Read the model definition and answer for the solid it produces. Units are mm, in the model's axes. Coordinates: 2 decimals unless noted, no trailing zeros. Write each loop counter-clockwise with the first axis right and the second up, starting at its lowest first coordinate (ties: lowest second). Pieces come first, ordered by that corner, then holes. Notation, with made-up numbers: (71, 61) - (101, 61) arc R22 cw to (101, 78) - close; hole circle Ø11 at (37.25, 31). An arc over 180 degrees is marked (long way). Use a Markdown table: item, result.
from build123d import *

# Parameters (mm, degrees)
SKETCH_1_W          = 381
SKETCH_1_H          = 110
EXTRUDE_1_DEPTH     = 5
SKETCH_2_R          = 2
CUT_EXTRUDE_1_DEPTH = 5
CUT_EXTRUDE_2_DEPTH = 5
SKETCH_6_R          = 1.5
CUT_EXTRUDE_3_DEPTH = 5
CUT_EXTRUDE_4_DEPTH = 10
FILLET_1_R          = 10


with BuildPart() as part:
    # 草图1 → 凸台-拉伸1 (new body)
    with BuildSketch(Plane.XY):
        with Locations((190.5, 55)):
            Rectangle(SKETCH_1_W, SKETCH_1_H)
    extrude(amount=EXTRUDE_1_DEPTH)

    # 草图2 → 切除-拉伸1 (cut)
    with BuildSketch(Plane.XY.offset(5)):
        with Locations((3.5, 105)):
            Circle(SKETCH_2_R)
        with Locations((3.5, 55)):
            Circle(SKETCH_2_R)
        with Locations((3.5, 5)):
            Circle(SKETCH_2_R)
        with Locations((377.5, 105)):
            Circle(SKETCH_2_R)
        with Locations((377.5, 55)):
            Circle(SKETCH_2_R)
        with Locations((377.5, 5)):
            Circle(SKETCH_2_R)
        with Locations((91.65, 105)):
            Circle(SKETCH_2_R)
        with Locations((91.65, 55)):
            Circle(SKETCH_2_R)
        with Locations((91.65, 5)):
            Circle(SKETCH_2_R)
        with Locations((289.35, 105)):
            Circle(SKETCH_2_R)
        with Locations((289.35, 55)):
            Circle(SKETCH_2_R)
        with Locations((289.35, 5)):
            Circle(SKETCH_2_R)
    extrude(amount=-CUT_EXTRUDE_1_DEPTH, mode=Mode.SUBTRACT)

    # 草图3 → 切除-拉伸2 (cut)
    with BuildSketch(Plane.XY.offset(5)):
        with BuildLine():
            Line((20, 100), (76.65, 100))
            ThreePointArc((76.65, 100), (83.721067812, 97.071067812), (86.65, 90))
            Line((86.65, 90), (86.65, 70))
            ThreePointArc((86.65, 70), (83.721067812, 62.928932188), (76.65, 60))
            Line((76.65, 60), (20, 60))
            ThreePointArc((20, 60), (12.928932188, 62.928932188), (10, 70))
            Line((10, 70), (10, 90))
            ThreePointArc((10, 90), (12.928932188, 97.071067812), (20, 100))
        make_face()
        with BuildLine():
            Line((20, 50), (76.65, 50))
            ThreePointArc((76.65, 50), (83.721067812, 47.071067812), (86.65, 40))
            Line((86.65, 40), (86.65, 20))
            ThreePointArc((86.65, 20), (83.721067812, 12.928932188), (76.65, 10))
            Line((76.65, 10), (20, 10))
            ThreePointArc((20, 10), (12.928932188, 12.928932188), (10, 20))
            Line((10, 20), (10, 40))
            ThreePointArc((10, 40), (12.928932188, 47.071067812), (20, 50))
        make_face()
        with BuildLine():
            Line((106.65, 100), (274.35, 100))
            ThreePointArc((274.35, 100), (281.421067812, 97.071067812), (284.35, 90))
            Line((284.35, 90), (284.35, 70))
            ThreePointArc((284.35, 70), (281.421067812, 62.928932188), (274.35, 60))
            Line((274.35, 60), (106.65, 60))
            ThreePointArc((106.65, 60), (99.578932188, 62.928932188), (96.65, 70))
            Line((96.65, 70), (96.65, 90))
            ThreePointArc((96.65, 90), (99.578932188, 97.071067812), (106.65, 100))
        make_face()
        with BuildLine():
            Line((106.65, 50), (274.35, 50))
            ThreePointArc((274.35, 50), (281.421067812, 47.071067812), (284.35, 40))
            Line((284.35, 40), (284.35, 20))
            ThreePointArc((284.35, 20), (281.421067812, 12.928932188), (274.35, 10))
            Line((274.35, 10), (106.65, 10))
            ThreePointArc((106.65, 10), (99.578932188, 12.928932188), (96.65, 20))
            Line((96.65, 20), (96.65, 40))
            ThreePointArc((96.65, 40), (99.578932188, 47.071067812), (106.65, 50))
        make_face()
        with BuildLine():
            Line((304.35, 100), (361, 100))
            ThreePointArc((361, 100), (368.071067812, 97.071067812), (371, 90))
            Line((371, 90), (371, 73))
            ThreePointArc((371, 73), (368.071067812, 65.928932188), (361, 63))
            Line((361, 63), (304.35, 63))
            ThreePointArc((304.35, 63), (297.278932188, 65.928932188), (294.35, 73))
            Line((294.35, 73), (294.35, 90))
            ThreePointArc((294.35, 90), (297.278932188, 97.071067812), (304.35, 100))
        make_face()
        with BuildLine():
            Line((304.35, 47), (361, 47))
            ThreePointArc((361, 47), (368.071067812, 44.071067812), (371, 37))
            Line((371, 37), (371, 20))
            ThreePointArc((371, 20), (368.071067812, 12.928932188), (361, 10))
            Line((361, 10), (304.35, 10))
            ThreePointArc((304.35, 10), (297.278932188, 12.928932188), (294.35, 20))
            Line((294.35, 20), (294.35, 37))
            ThreePointArc((294.35, 37), (297.278932188, 44.071067812), (304.35, 47))
        make_face()
    extrude(amount=-CUT_EXTRUDE_2_DEPTH, mode=Mode.SUBTRACT)

    # 草图6 → 切除-拉伸3 (cut)
    with BuildSketch(Plane(origin=(0, 0, 0), x_dir=(-1, 0, 0), z_dir=(0, 0, -1))):
        with Locations((-361, 60)):
            Circle(SKETCH_6_R)
        with Locations((-351, 60)):
            Circle(SKETCH_6_R)
        with Locations((-361, 50)):
            Circle(SKETCH_6_R)
        with Locations((-351, 50)):
            Circle(SKETCH_6_R)
    extrude(amount=-CUT_EXTRUDE_3_DEPTH, mode=Mode.SUBTRACT)

    # 草图7 → 切除-拉伸4 (cut)
    with BuildSketch(Plane.XY.offset(5)):
        Polygon((96.65, 90), (96.65, 100), (284.35, 100), (284.35, 10), (96.65, 10), align=None)
    extrude(amount=-CUT_EXTRUDE_4_DEPTH, mode=Mode.SUBTRACT)

    # 圆角1
    fillet_1_edges = [part.edges().sort_by_distance(p)[0] for p in [
        (96.65, 100, 2.5),
        (96.65, 10, 2.5),
        (284.35, 100, 2.5),
        (284.35, 10, 2.5),
    ]]
    fillet(fillet_1_edges, radius=FILLET_1_R)


solid = part.part
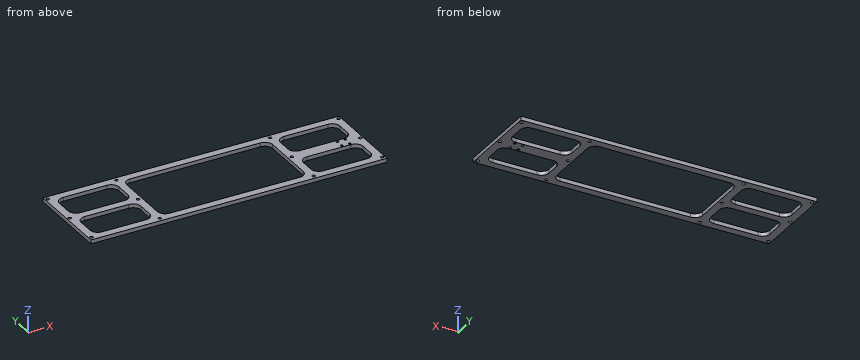
(1) Straight lines are drawn through the part: L1, parallel to X at y = 5.5, z = 0.6; L2, parallel to X at y = 35, z = 2.2; L3, parallel to Y at x = 25, z = 0.85. For each, find the intervals that lie inside material, in ascending order.
Report:
| item | result |
|---|---|
| L1 | x = 0 to 1.56, 5.44 to 89.71, 93.59 to 287.41, 291.29 to 375.56, 379.44 to 381 |
| L2 | x = 0 to 10, 86.65 to 96.65, 284.35 to 294.35, 371 to 381 |
| L3 | y = 0 to 10, 50 to 60, 100 to 110 |
(2) A cutting plane is placed at A-A, the plane x = 313. Write down the section's boundary in (y, z), and give its area (3 significant figures).
Report:
| item | result |
|---|---|
| outline | (0, 0) - (10, 0) - (10, 5) - (0, 5) - close; (47, 0) - (63, 0) - (63, 5) - (47, 5) - close; (100, 0) - (110, 0) - (110, 5) - (100, 5) - close |
| area | 180 mm² |
(3) A cutting plane is placed at B-B, the plane z = 2.25. Count the separate pieces of the cut face and the enclosed holes in it, and give its area (3 significant figures).
Report:
| item | result |
|---|---|
| separate pieces | 1 |
| enclosed holes | 21 |
| area | 13,500 mm² |
(4) This flat-tipped pin is pushed along its axis until it touches: P1, Ø3.5, axis at x = 361, y = 60, coming from the +Z side. Where does it stop, or does it pass through?
Report:
| item | result |
|---|---|
| P1 | stops at z = 5 |
